Part model, mm, in its own coordinate system. Face numbers are marked on the shaded views. A direction names the side the tool comes from. Round coordinates to 2 decimals unless told otherwise and drop trailing zeros. Order: outer loops, then holes, each group sorted by start corner. A loop starts at its lowest first (then second) coordinate and runs counter-clockwise, first axis right, second up. Notation, with made-up numbers: (15.25, 14.25) -> (38.25, 14.25) arc R29 cw to (38.25, 51.25) -> close; hole circle Ø6 at (-31, 28). An arc over 180 degrees is marked (long way). Answer as a JSON object with one key per item and string values. Group by question number.
```python
from build123d import *

# Parameters (mm, degrees)
F0_W      = 99.06
F0_H      = 101.6
F1_DEPTH  = 45.72
F2_W      = 38.1
F2_H      = 101.6
F3_DEPTH  = 35.56
F4_W      = 45.72
F4_H      = 66.04
F5_DEPTH  = 50.8
F6_R      = 7.9375
F7_DEPTH  = 101.601
F8_R      = 5.1562
F9_DEPTH  = 60.961
F10_R     = 5.1562
F11_DEPTH = 10.161
F12_R     = 10.16


with BuildPart() as f1:
    # F0 (on Front) → F1 (new body)
    with BuildSketch(Plane.XZ):
        with Locations((49.53, 50.8)):
            Rectangle(F0_W, F0_H)
    extrude(amount=F1_DEPTH)

    # F2 (on face) → F3 (cut)
    with BuildSketch(Plane.XZ.offset(45.72)):
        with Locations((80.01, 50.8)):
            Rectangle(F2_W, F2_H)
    extrude(amount=-F3_DEPTH, mode=Mode.SUBTRACT)

    # F4 (on face) → F5 (cut)
    with BuildSketch(Plane(origin=(0, 0, 0), x_dir=(0, -1, 0), z_dir=(-1, 0, 0))):
        with Locations((22.86, 50.8)):
            Rectangle(F4_W, F4_H)
    extrude(amount=-F5_DEPTH, mode=Mode.SUBTRACT)

    # F6 (on face) → F7 (cut, through all)
    with BuildSketch(Plane.XY.offset(101.6)):
        with Locations((22.86, -22.86)):
            Circle(F6_R)
        with BuildLine():
            ThreePointArc((0, -22.86), (6.6955389909, -6.6955389733), (22.8600000249, 0))
            Line((22.8600000249, 0), (0, 0))
            Line((0, 0), (0, -22.86))
        make_face()
        with BuildLine():
            Line((0, -45.72), (22.86, -45.72))
            ThreePointArc((22.86, -45.72), (6.6955389821, -39.0244610179), (0, -22.86))
            Line((0, -22.86), (0, -45.72))
        make_face()
    extrude(amount=-F7_DEPTH, mode=Mode.SUBTRACT)

    # F8 (on face) → F9 (cut, through all)
    with BuildSketch(Plane.YZ.offset(60.96)):
        with Locations((-27.94, 50.8)):
            Circle(F8_R)
    extrude(amount=-F9_DEPTH, mode=Mode.SUBTRACT)

    # F10 (on face) → F11 (cut, through all)
    with BuildSketch(Plane.XZ.offset(10.16)):
        with Locations((80.01, 86.36)):
            Circle(F10_R)
        with Locations((80.01, 15.24)):
            Circle(F10_R)
    extrude(amount=-F11_DEPTH, mode=Mode.SUBTRACT)

    # F12
    f12_edges = [f1.edges().sort_by_distance(p)[0] for p in [
        (99.06, -5.08, 101.6),
        (99.06, -5.08, 0),
    ]]
    fillet(f12_edges, radius=F12_R)


solid = f1.part
```
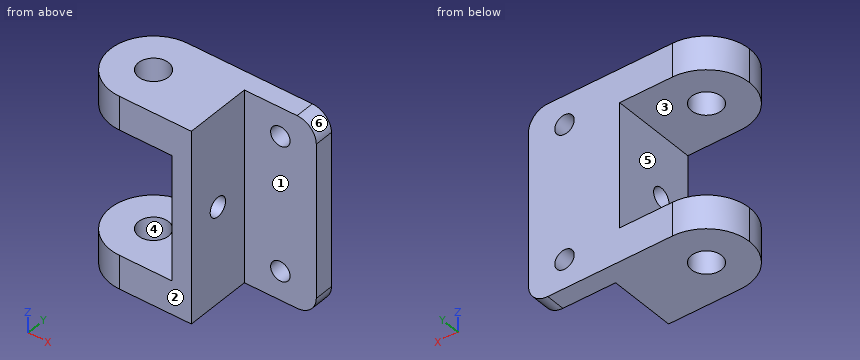
Q1. Band-saw the part on C-C (z = 50.8). List the corners of the cut face in (x, y), plus the area to 3 significant figures.
Q2. Two-plate mould, pull along X, no slides. Class the marked faces 4, 5 and 6: +X half, -X half, draft (parallel to the pull), parting line (faces both ways), or undercut.
Q3. Drop flat-ended pins along their axis: pin 1 Ø10 at (y, z) = (-24, 62.5) entering from +X; pin 2 Ø13.5 at (y, z) = (-32, 57.5) entering from -X; pin 3 Ø19 at (x, z) = (76.5, 72.5) entering from -Y; pin 4 Ø2 at (x, y) = (29, -12.5) entering from -Z. Give the stop position or say it passes through.
Q4. Band-saw the part on B-B (x = 80.01). List the corners of the cut face in (y, z), plus the area to 3 significant figures.
Q5. Band-saw the part on D-D (y = -27.94). List the corners of the cut face in (x, z).
Q6. Wall check: line 1 (Z direction, x = 80.01, y = -3.75); line 2 (Z direction, x = 45, y = -42); line 3 (Z direction, x = 57.25, y = -27.94). Give the ranges that are in metal, low to high. Write a range as [from, to].
Q7. Which spindle directions (+Z, -Z, +X, -X, +Y, -Y) get a long thin tool onto all of the face, cutting with end or side? Do the marked faces 1, 2 and 3. Say none if no direction does.
Completed:
{
 "1": {"outline": "(50.8, -45.72) -> (60.96, -45.72) -> (60.96, -33.1) -> (50.8, -33.1) -> close; (50.8, -22.78) -> (60.96, -22.78) -> (60.96, -10.16) -> (99.06, -10.16) -> (99.06, 0) -> (50.8, 0) -> close", "area": "747 mm2"},
 "2": {"face 4": "undercut", "face 5": "-X half", "face 6": "+X half"},
 "3": {"pin 1": "x = 60.96", "pin 2": "x = 50.8", "pin 3": "y = -10.16", "pin 4": "z = 0"},
 "4": {"outline": "(-10.16, 0) -> (0, 0) -> (0, 10.08) -> (-10.16, 10.08) -> close; (-10.16, 20.4) -> (0, 20.4) -> (0, 81.2) -> (-10.16, 81.2) -> close; (-10.16, 91.52) -> (0, 91.52) -> (0, 101.6) -> (-10.16, 101.6) -> close", "area": "823 mm2"},
 "5": {"outline": "(0.57, 0) -> (16.76, 0) -> (16.76, 17.78) -> (0.57, 17.78) -> close; (0.57, 83.82) -> (16.76, 83.82) -> (16.76, 101.6) -> (0.57, 101.6) -> close; (28.96, 0) -> (60.96, 0) -> (60.96, 45.64) -> (50.8, 45.64) -> (50.8, 17.78) -> (28.96, 17.78) -> close; (28.96, 83.82) -> (50.8, 83.82) -> (50.8, 55.96) -> (60.96, 55.96) -> (60.96, 101.6) -> (28.96, 101.6) -> close"},
 "6": {"line 1": "[0, 10.08], [20.4, 81.2], [91.52, 101.6]", "line 2": "[0, 17.78], [83.82, 101.6]", "line 3": "[0, 45.64], [55.96, 101.6]"},
 "7": {"face 1": "+Z, -Z, +X, -Y", "face 2": "+Z, -Z, +X, -X, -Y", "face 3": "-X, +Y, -Y"}
}
